Autodesk Inventor part; units mm, degrees
ref_plane "YZ Plane" through (0, 0, 0) normal (1, 0, 0) x (0, 1, 0)
ref_plane "XZ Plane" through (0, 0, 0) normal (0, 1, 0) x (-1, 0, 0)
ref_plane "XY Plane" through (0, 0, 0) normal (0, 0, 1) x (1, 0, 0)
sketch "Esquisse1" plane through (0, 0, 0) normal (0, 0, 1) x (1, 0, 0)
  point P0 (0, 0)
sketch "Esquisse2" plane through (0, 0, 0) normal (0, 0, 1) x (1, 0, 0)
  line L0 (0, 0) -> (156, 0)
  line L1 (0, 46.8) -> (0, 0)
  line L2 (194.0737, 12.2634) -> (156, 0)
  arc A0 (194.0737, 12.2634) -> (194.0737, 34.5366) centre (190.4867, 23.4) ccw
  line L3 (0, 46.8) -> (156, 46.8)
  line L4 (156, 46.8) -> (194.0737, 34.5366)
  dimension "d0" = 156
  dimension "d1" = 46.8
  dimension "d2" = 11.7
  dimension "d4" = 40
  dimension "d6" = 40
extrude "Extrusion1" add sketch "Esquisse2" along normal blind 5
sketch "Esquisse3" plane through (0, 0, 5) normal (0, 0, 1) x (1, 0, 0)
  line L0 (194.0737, 34.5366) -> (156, 46.8)
  line L1 (156, 46.8) -> (156, 0)
  circle A0 centre (156, 23.4) radius 5
  point P0 (0, 0)
  dimension "d11" = 23.4
  dimension "d12" = 10
extrude "Extrusion2" cut sketch "Esquisse3" against normal blind 5
sketch "Esquisse4" plane through (0, 0, 5) normal (0, 0, 1) x (1, 0, 0)
  point P0 (0, 0)
sketch "Esquisse5" plane through (0, 0, 5) normal (0, 0, 1) x (1, 0, 0)
  arc A0 (194.0737, 12.2634) -> (194.0737, 34.5366) centre (190.4867, 23.4) ccw
  circle A1 centre (190.4867, 23.4) radius 3
  point P0 (0, 0)
  point P1 (194.0737, 12.2634)
  dimension "d17" = 6
extrude "Extrusion3" add sketch "Esquisse5" along normal blind 5
sketch "Esquisse6" plane through (190.4867, 23.4, 10) normal (0, 0, 1) x (1, 0, 0)
  circle A0 centre (0, 0) radius 1.5
  point P0 (-190.4867, -23.4)
  dimension "d20" = 3
extrude "Extrusion4" cut sketch "Esquisse6" against normal blind 5
sketch "Esquisse7" plane through (0, 0, 0) normal (-1, 0, 0) x (0, 0, 1)
  line L0 (0, 0) -> (-63.96, 0)
  line L1 (-63.96, 0) -> (-63.96, 46.8)
  line L2 (-63.96, 46.8) -> (0, 46.8)
  line L3 (0, 46.8) -> (0, 0)
  dimension "d23" = 63.96
  dimension "d24" = 46.8
extrude "Extrusion5" add sketch "Esquisse7" against normal blind 5
sketch "Esquisse8" plane through (0, 0, 5) normal (-1, 0, 0) x (0, 0, 1)
  line L0 (-68.96, 46.8) -> (0, 46.8)
  line L1 (-68.96, 46.8) -> (0, 0)
  line L2 (0, 46.8) -> (-68.96, 0)
  circle A0 centre (-34.48, 23.4) radius 7
  point P0 (-5, 0)
  dimension "d27" = 14
extrude "Extrusion6" add sketch "Esquisse8" along normal blind 2 contours A0 L2 L1 | L1 L2 A0 | A0 L1 L2 | L1 A0 L2
sketch "Esquisse9" plane through (-2, 23.4, -29.48) normal (-1, 0, 0) x (0, 0, 1)
  circle A0 centre (0, 0) radius 5
  point P0 (29.48, -23.4)
  dimension "d30" = 10
extrude "Extrusion7" cut sketch "Esquisse9" against normal blind 7
sketch "Esquisse10" plane through (0, 0, -63.96) normal (0, 0, -1) x (-1, 0, 0)
  line L0 (-5, 0) -> (-5, 46.8)
  line L1 (-5, 46.8) -> (-156, 46.8)
  line L2 (-156, 0) -> (-5, 0)
  line L3 (-5, 0) -> (-5, 46.8)
  arc A0 (-156, 46.8) -> (-156, 0) centre (-156, 23.4) ccw
  point P0 (0, 0)
  dimension "d33" = 151
extrude "Extrusion8" add sketch "Esquisse10" against normal blind 5
sketch "Esquisse11" plane through (0, 0, -63.96) normal (0, 0, -1) x (-1, 0, 0)
  arc A0 (-156, 46.8) -> (-156, 0) centre (-156, 23.4) ccw
  circle A1 centre (-156, 23.4) radius 5
  point P0 (0, 0)
  dimension "d36" = 10
extrude "Extrusion9" cut sketch "Esquisse11" against normal blind 5
ref_plane "Plan de construction1" through (115.24, 0, 0) normal (1, 0, 0) x (0, 0, -1)
sketch "Esquisse12" plane through (115.24, 0, 0) normal (1, 0, 0) x (0, 0, -1)
  line L0 (0, 0) -> (0, 13)
  line L1 (0, 0) -> (0, 46.8)
  line L2 (0, 13) -> (2, 13)
  line L3 (0, 0) -> (58.96, 0)
  line L4 (58.96, 0) -> (58.96, 46.8)
  line L5 (12, 23) -> (12, 31.8)
  line L6 (27, 46.8) -> (58.96, 46.8)
  arc A0 (2, 13) -> (12, 23) centre (2, 23) ccw
  arc A1 (27, 46.8) -> (12, 31.8) centre (27, 31.8) ccw
  point P0 (12, 13)
  dimension "d40" = 13
  dimension "d41" = 12
  dimension "d42" = 46.8
  dimension "d44" = 10
  dimension "d45" = 15
extrude "Extrusion10" add sketch "Esquisse12" along normal blind 5
fillet "Congé1" radius 2 4 edges at (120.24, 6.5, 0) (120.24, 23.4, -58.96) (115.24, 23.4, -58.96) (115.24, 6.5, 0)
fillet "Congé2" radius 2 2 edges at (5, 23.4, 0) (5, 23.4, -58.96)
sketch "Esquisse13" plane through (120.24, 0, 0) normal (1, 0, 0) x (0, 0, -1)
  line L0 (63.96, 46.8) -> (-5, 46.8)
  line L1 (0, 46.8) -> (58.706, 0)
  line L2 (58.706, 46.8) -> (0, 0)
  circle A0 centre (29.353, 23.4) radius 7
  dimension "d51" = 14
extrude "Extrusion11" add sketch "Esquisse13" along normal blind 2 contours A0 L1 L2 | L2 L1 A0 | L1 L2 A0 | L1 A0 L2
sketch "Esquisse14" plane through (122.24, 23.4, -29.353) normal (1, 0, 0) x (0, 0, -1)
  circle A0 centre (0, 0) radius 5
  point P0 (-29.353, -23.4)
  dimension "d54" = 10
extrude "Extrusion12" cut sketch "Esquisse14" against normal blind 7
properties part number "Right forearm" material "Plastique ABS"
Design review of the part built by this model. Coordinates are the model's own, in mm. A direction names the side the tool comes from. Give positions to 0.01 mm unless a question says otherwise; leave off trailing zeros. Loops run counter-clockwise (first coordinate to the right, second up) from the corner with the lowest first, then second, coordinate; pieces in that order, holes last. Notation, with made-up numbers: M 73,-21 L 117,-21 A23 cw 117,2 Z; hole C 78,34 d3. An arc over 180 degrees is marked long. Write item = value, one per line.
Q1. Insertion check: pin 1 (10 mm diameter, centred on y = 25, z = -10.5, fed in from -X); pin 2 (2 mm diameter, centred on x = 169.5, y = 15, fed in from +Z); pin 3 (14 mm diameter, centred on y = 29.5, z = -22, fed in from +X). Each pin has a flat end and moves straight along its axis. Give the tip position at first contact, or say it passes through.
Output values:
pin_1 = 0
pin_2 = 5
pin_3 = 122.24
Q2. To check wall thickness, follow line 1 (Y direction, x = 156, z = -62.1); line 2 (Z direction, x = 36.5, y = 10.5); line 3 (X direction, y = 23, z = -61). State the ranges of each line that lie inside material, in increasing order. Write a range as [from, to].
Output values:
line_1 = [0, 18.4], [28.4, 46.8]
line_2 = [-63.96, -58.96], [0, 5]
line_3 = [0, 151.02], [160.98, 179.4]
Q3. Draft analysis for pull direction Z (two halves, no side actions). For faces 5 (the cylindrical face through (202.185, 23.606, 2.465)), 6 (the flat face through (118, 27, -12)), 7 (the flat face through (191, 25, 10)), state which applies: +Z half, -Z half, draft (parallel to the pull), parting line (faces both ways), or undercut.
Output values:
face_5 = draft
face_6 = undercut
face_7 = +Z half
Q4. For faces 1 (the cylindrical face through (121.23, 17.5, -33.12)), 2 (the flat face through (175.303, 6.218, 2.465)), 3 (the flat face through (61, 24, -58.96)), 4 (the cylindrical face through (-0.986, 21.297, -22.803)), list the 3-axis set-ups (+Z, -Z, +X, -X, +Y, -Y) from which the entire face can be reached by the end or side of a thin tool; tool diameter is ignored.
Output values:
face_1 = +X
face_2 = +Z, +X, -Y
face_3 = +Y, -Y
face_4 = -X
Q5. We need section C-C (y = 9). Give the boundary of the cut face in (x, z), plus the area to 3 significant figures.
Output values:
outline = M 0,-63.96 L 174.44,-63.96 L 174.44,-58.96 L 122.24,-58.96 A2 cw 120.24,-56.96 L 120.24,-2 A2 cw 122.24,0 L 183.94,0 L 183.94,5 L 0,5 Z; hole M 5,-56.96 A2 ccw 7,-58.96 L 113.24,-58.96 A2 ccw 115.24,-56.96 L 115.24,-2 A2 ccw 113.24,0 L 7,0 A2 ccw 5,-2 Z
area = 2,390 mm^2
Q6. We need section A-A (x = 73.5). Give the boundary of the cut face in (y, z).
Output values:
outline = M 0,-63.96 L 46.8,-63.96 L 46.8,-58.96 L 0,-58.96 Z; M 0,0 L 46.8,0 L 46.8,5 L 0,5 Z
Q7. We need section B-B (z = -14.5). Give the boundary of the cut face in (x, y).
Output values:
outline = M 0,0 L 5,0 L 5,46.8 L 0,46.8 Z; M 115.24,0 L 120.24,0 L 120.24,40.09 L 115.24,40.09 Z
